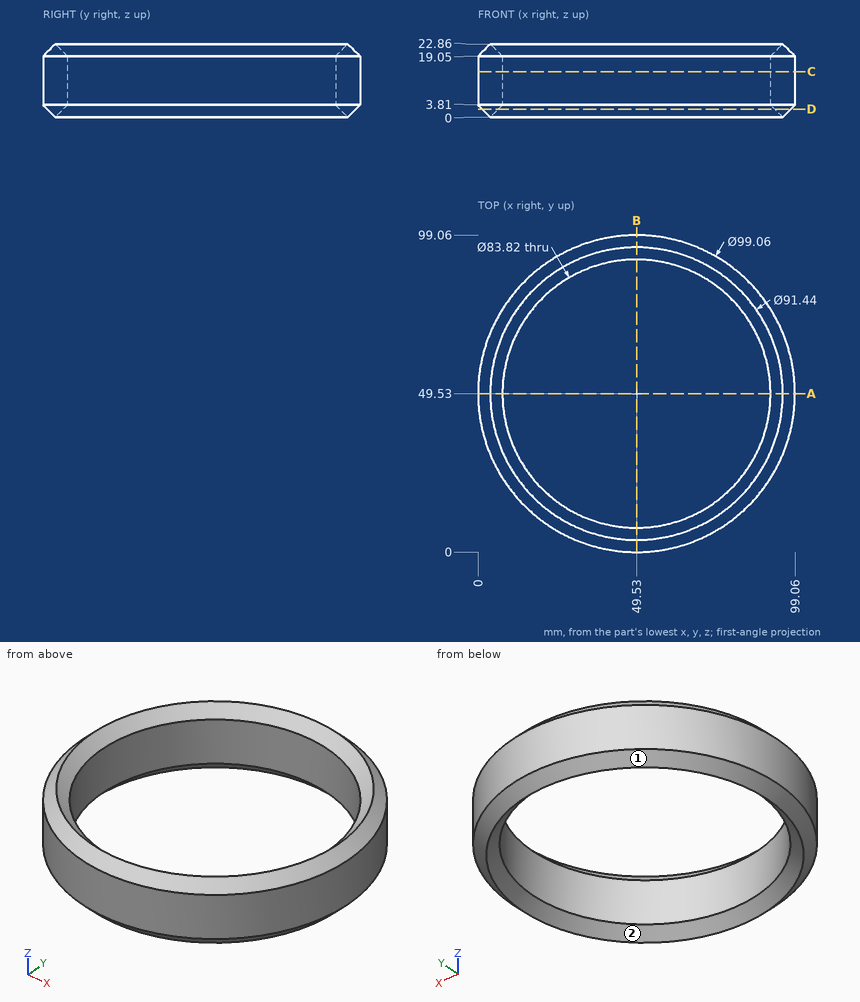
Here's the drawing with two shaded views (mm, measured from the low corner). I have some questions. Round coordinates to 2 decimals unless told otherwise and drop trailing zeros. Write each loop counter-clockwise with the first axis right and the second up, starting at its lowest first coordinate (ties: lowest second). Pieces come first, ordered by that corner, then holes. Notation, with made-up numbers: M 9.25,53.5 L 14.25,53.5 A27 cw 14.25,69.5 Z; hole C -26,-9.75 d7. An arc over 180 degrees is marked long. Use CSV: the item, a comma, the result in double quotes.
(1) Imagine slicing it at C-C (z = 14.25). Write out the boundary of the cut face in (x, y), plus the area to 3 significant figures.
Check values:
outline,"C 49.53,49.53 d99.06; hole C 49.53,49.53 d83.82"
area,"2,190 mm^2"
(2) We'd pull the mould along Y, two halves only. Please class the marked faces 1 and 2: +Y half, -Y half, draft (parallel to the pull), parting line (faces both ways), or undercut.
Check values:
face 1,"parting line"
face 2,"undercut"
(3) Imagine slicing it at D-D (z = 2.5). Write out the boundary of the cut face in (x, y), plus the area to 3 significant figures.
Check values:
outline,"C 49.53,49.53 d96.44; hole C 49.53,49.53 d86.44"
area,"1,440 mm^2"
(4) I need wall thicknesses on line 1 along Y through (x, z) = (49.53, 9.5); line 2 along X through (y, z) = (46.5, 15.25); line 3 along Y through (x, z) = (80.5, 18.5). Which ranges of each line are inside material? Lowest first, please.
Check values:
line 1,"0 to 7.62, 91.44 to 99.06"
line 2,"0.09 to 7.73, 91.33 to 98.97"
line 3,"10.88 to 21.29, 77.77 to 88.18"
(5) I'm going to push flat-ended pins straight in: pin 1 (1.5 mm diameter, centred on x = 81.5, z = 6.5, fed in from +Y); pin 2 (1.5 mm diameter, centred on x = 83.5, y = 84, fed in from -Z); pin 3 (12 mm diameter, centred on x = 51.5, z = 14, fed in from +Y). Where does each tip first touch, or does it pass through?
Check values:
pin 1,"y = 87.98"
pin 2,"z = 1.93"
pin 3,"y = 99.06"
(6) Imagine slicing it at A-A (y = 49.53). Write out the boundary of the cut face in (x, z).
Check values:
outline,"M 0,3.81 L 3.81,0 L 7.62,3.81 L 7.62,19.05 L 3.81,22.86 L 0,19.05 Z; M 91.44,3.81 L 95.25,0 L 99.06,3.81 L 99.06,19.05 L 95.25,22.86 L 91.44,19.05 Z"
